Can you work these out from the model? Positions are in its coordinate system, mm. A direction names the side the tool comes from. Coordinates: 2 decimals unless noted, no trailing zeros. Order: outer loops, then holes, each group sorted by start corner. A loop starts at its lowest first (then second) coordinate and runs counter-clockwise, first axis right, second up. Notation, with made-up numbers: (-3.75, 5.5) -> (33.25, 5.5) arc R14 cw to (33.25, 18.5) -> close; hole circle Ø2 at (-22.75, 84). An arc over 180 degrees is marked (long way). Answer in a Markdown table with one row per item. Add a question column.
1. We'd pull the mould along Z, two halves only. Please class faces 3 (the face through (-5.963, -0.063, -0.663)), 4 (the face through (74, 0, 2)), 5 (the face through (0, 0, -2)): pulls with the +Z half, pulls with the -Z half, needs draft (parallel to the pull), parting line crosses it, or undercut.
2. Imagine slicing it at D-D on x = 60. Write out the boundary of the cut face in (y, z).
3. Will these pins go through, and if not, where does the flat tip stop? pin 1 (1.5 mm diameter, centred on y = 0.5, z = -3, fed in from +X); pin 2 (4.5 mm diameter, centred on x = 60, y = 0, fed in from -Z); pin 3 (4 mm diameter, centred on x = 5, y = -1, fed in from +Z).
4. Imagine slicing it at A-A on z = 0. State how many separate pieces and enclosed holes the cut face has, plus the area to 3 significant figures.
5. On a 3-axis mill with a long thin cutter (end or side, diameter ignored), from which of +Z, -Z, +X, -X, +Y, -Y can I reach the whole of each face in a straight line? I mean faces 1 (the face through (65.253, 0.121, 5.481)), 2 (the face through (35, 0, 9)). Say none if no direction works.
6. If I drill on line 1 along X through (y, z) = (-2, 0.25); line 2 along Z through (x, y) = (33, -1.25); line 3 along Z through (x, y) = (-1, 2), over which ranges is the centre line in solid material (lowest first)? Write a range as [from, to].
7. Imagine slicing it at B-B on x = 23. Write out the boundary of the cut face in (y, z), plus the area to 4 significant figures.
from build123d import *

# Parameters (mm, degrees)
F0_R           = 2
F0_R_2         = 1.5
F1_DEPTH       = 4.5
F2_R           = 2
F3_R           = 20
F4_SIZE        = 0.5
F6_D           = 3.5
F6_CBORE_D     = 5.5
F6_CBORE_DEPTH = 4.9


with BuildPart() as f1:
    # F0 (on Front) → F1 (new body, symmetric)
    with BuildSketch(Plane.XZ):
        with BuildLine():
            Line((10.406237, 9), (-1.552914, 5.795555))
            ThreePointArc((-1.552914, 5.795555), (-5.948669, -0.783157), (0, -6))
            Line((0, -6), (54, -6))
            Line((54, -6), (54, -1))
            Line((54, -1), (74, -1))
            Line((74, -1), (74, 6))
            Line((74, 6), (56.986155, 9))
            Line((56.986155, 9), (10.406237, 9))
        make_face()
        Circle(F0_R, mode=Mode.SUBTRACT)
        with Locations((23, 0)):
            Circle(F0_R_2, mode=Mode.SUBTRACT)
        with Locations((33, 0)):
            Circle(F0_R_2, mode=Mode.SUBTRACT)
    extrude(amount=F1_DEPTH, both=True)

    # F2
    f2_edges = [f1.edges().sort_by_distance(p)[0] for p in [
        (74, 0, 6),
    ]]
    fillet(f2_edges, radius=F2_R)

    # F3
    f3_edges = [f1.edges().sort_by_distance(p)[0] for p in [
        (10.406237, 0, 9),
    ]]
    fillet(f3_edges, radius=F3_R)

    # F4
    f4_edges = [f1.edges().sort_by_distance(p)[0] for p in [
        (-2, -4.5, 0),
        (21.5, -4.5, 0),
        (31.5, -4.5, 0),
        (-2, 4.5, 0),
        (21.5, 4.5, 0),
        (31.5, 4.5, 0),
    ]]
    chamfer(f4_edges, length=F4_SIZE)

    # F6 (through all)
    with Locations(Plane.XY.offset(9)):
        with Locations((60, 0), (68, 0)):
            CounterBoreHole(F6_D / 2, F6_CBORE_D / 2, F6_CBORE_DEPTH)


solid = f1.part
Answers follow:
| question | item | result |
|---|---|---|
| 1 | face 3 | parting line crosses it |
| 1 | face 4 | needs draft |
| 1 | face 5 | undercut |
| 2 | outline | (-4.5, -1) -> (-1.75, -1) -> (-1.75, 4.1) -> (-2.75, 4.1) -> (-2.75, 8.47) -> (-4.5, 8.47) -> close; (1.75, -1) -> (4.5, -1) -> (4.5, 8.47) -> (2.75, 8.47) -> (2.75, 4.1) -> (1.75, 4.1) -> close |
| 3 | pin 1 | stops at x = 54 |
| 3 | pin 2 | stops at z = -1 |
| 3 | pin 3 | stops at z = 8.09 |
| 4 | separate pieces | 4 |
| 4 | enclosed holes | 2 |
| 4 | area | 609 mm² |
| 5 | face 1 | +Z |
| 5 | face 2 | +Z, +X, -X, +Y, -Y |
| 6 | line 1 | x = [-5.99, -1.98], [1.98, 21.52], [24.48, 31.52], [34.48, 74] |
| 6 | line 2 | z = [-6, -1.5], [1.5, 9] |
| 6 | line 3 | z = [-5.92, -1.73], [1.73, 5.94] |
| 7 | outline | (-4.5, -6) -> (4.5, -6) -> (4.5, -2) -> (4, -1.5) -> (-4, -1.5) -> (-4.5, -2) -> close; (-4.5, 2) -> (-4, 1.5) -> (4, 1.5) -> (4.5, 2) -> (4.5, 9) -> (-4.5, 9) -> close |
| 7 | area | 107.5 mm² |
